```python
from build123d import *
from build123d.topology import SkipClean

# Parameters (mm, degrees)
EXTRUDE_1_DEPTH     = 4
EXTRUDE_START       = -11
SKETCH_3_R          = 9
EXTRUDE_2_DEPTH     = 11
SKETCH_4_R          = 3
CUT_EXTRUDE_1_DEPTH = 50.484262082
HOLE_WIZARD_M4_1_D  = 3.3
SKETCH_10_R         = 6
CUT_EXTRUDE_2_DEPTH = 10
SKETCH_11_R         = 5.5
CUT_EXTRUDE_3_DEPTH = 50.484262082
SCALE1_SCALE        = 2


with BuildPart() as part:
    # 草图1 → 凸台-拉伸1 (new body)
    with BuildSketch(Plane(origin=(0, 0, 0), x_dir=(1, 0, 0), z_dir=(0, 1, 0))):
        with BuildLine():
            Line((-8.109776452, 3.902758754), (-25.406517635, -32.039176982))
            ThreePointArc((-25.406517635, -32.039176982), (-23, -39.837168574), (-15.043482365, -38.022278184))
            Line((-15.043482365, -38.022278184), (0.302963304, -15.526261061))
            Line((0.302963304, -15.526261061), (7.351564548, -25.039059461))
            ThreePointArc((7.351564548, -25.039059461), (12.25592959, -26.282925824), (14.455537758, -21.72642235))
            Line((14.455537758, -21.72642235), (8.752682732, 2.095362733))
            ThreePointArc((8.752682732, 2.095362733), (0.95916746, 8.948742805), (-8.109776452, 3.902758754))
        make_face()
    extrude(amount=EXTRUDE_1_DEPTH)

    # 草图3 → 凸台-拉伸2 (add)
    with SkipClean():  # the faces are left unmerged after this step: merging them gives an invalid solid
        with BuildSketch(Plane(origin=(0, 4, 0), x_dir=(1, 0, 0), z_dir=(0, 1, 0)).offset(EXTRUDE_START)):
            with Locations(Location((0, 0, 0), (0, 0, 154.301222305))):
                Circle(SKETCH_3_R)
        extrude(amount=EXTRUDE_2_DEPTH)

    # 草图4 → 切除-拉伸1 (cut, through all)
    with SkipClean():  # the faces are left unmerged after this step: merging them gives an invalid solid
        with BuildSketch(Plane(origin=(0, 4, 0), x_dir=(1, 0, 0), z_dir=(0, 1, 0))):
            with Locations(Location((-20, -34.641016151, 0), (0, 0, 270))):
                Circle(SKETCH_4_R)
        extrude(amount=-CUT_EXTRUDE_1_DEPTH, mode=Mode.SUBTRACT)

    # M4 螺纹孔1 (through all)
    with Locations(Plane(origin=(0, 4, 0), x_dir=(1, 0, 0), z_dir=(0, 1, 0))):
        with Locations((10.565456544, -22.657694676)):
            Hole(HOLE_WIZARD_M4_1_D / 2)

    # 草图10 → 切除-拉伸2 (cut)
    with SkipClean():  # the faces are left unmerged after this step: merging them gives an invalid solid
        with BuildSketch(Plane(origin=(0, 4, 0), x_dir=(1, 0, 0), z_dir=(0, 1, 0))):
            with Locations(Location((0, 0, 0), (0, 0, 270))):
                Circle(SKETCH_10_R)
        extrude(amount=-CUT_EXTRUDE_2_DEPTH, mode=Mode.SUBTRACT)

    # 草图11 → 切除-拉伸3 (cut, through all)
    with SkipClean():  # the faces are left unmerged after this step: merging them gives an invalid solid
        with BuildSketch(Plane.XZ.offset(7)):
            with Locations(Location((0, 0, 0), (0, 0, 270))):
                Circle(SKETCH_11_R)
        extrude(amount=-CUT_EXTRUDE_3_DEPTH, mode=Mode.SUBTRACT)


with BuildPart() as part_1:
    # Scale1: scaled about (-4.168101576, 0.704724682, 12.285042226)
    add(part.part.scale(SCALE1_SCALE).moved(Location((4.168101576, -0.704724682, -12.285042226))))


solid = part_1.part
```
CAD build for the part. Positions are in the model's coordinates, mm. A direction names the side the tool comes from. Round coordinates to 2 decimals unless told otherwise and drop trailing zeros. Order: outer loops, then holes, each group sorted by start corner. A loop starts at its lowest first (then second) coordinate and runs counter-clockwise, first axis right, second up.
Q1. Slice it at B-B (x = -2). Write the cut outline in (y, z), and give its area (3 significant figures).
Q2. Which spindle directions (+Z, -Z, +X, -X, +Y, -Y) get a long thin tool onto all of the face, cutting with end or side? Do faces 1 (the flat face through (11.724, 3.239, 28.147)), 2 (the flat face through (15, -14.705, -16)), 3 (the flat face through (-6, -12.705, -7)). Say none if no direction does.
Q3. Slice it at D-D (z = 2). Write the cut outline in (x, y).
Q4. Two-plate mould, pull along Z, no slides. Class faces 4 (the flat face through (-8, -0.705, 24)), 5 (the cylindrical face through (-34.03, 3.35, 62.72)), 6 (the flat face through (27.456, 3.239, 7.68)): pulls with the +Z half, pulls with the -Z half, needs draft (parallel to the pull), parting line crosses it, or undercut.
Q5. Wall check: L1, parallel to Y at x = -6, z = 27; L2, parallel to X at y = -3.5, z = -12.5; L3, parallel to X at y = -13, z = -2.5. Give the ranges that are in metal, low to high.
Q6. Slice it at C-C (y = 5.5). Write the cut outline in (x, z), and give its area (3 significant figures).
Q7. Slice it at A-A (z = -11.5). Write the cut outline in (x, y).
Q8. Drop flat-ended pins along their axis: pin 1 (1.5 mm diameter, centred on x = 4, y = 2.5, fed in from +Z); pin 2 (11 mm diameter, centred on x = -35.83, z = 57, fed in from -Y); pin 3 (2 mm diameter, centred on x = 22, z = 20, fed in from -Y). Give the stop position or say it passes through.
Results below:
1. outline: (-14.7, -29.2) - (7.3, -29.2) - (7.3, -22.58) - (-12.7, -22.58) - (-12.7, -21.39) - (-14.7, -21.39) - close; (-14.7, -3.18) - (-12.7, -3.18) - (-12.7, -1.99) - (7.3, -1.99) - (7.3, 28.7) - (-0.7, 28.7) - (-0.7, 4.63) - (-14.7, 4.63) - close
1. area: 488 mm2
2. face 1: +Z, +Y, -Y
2. face 2: +Z, -Z, +X, -X, -Y
2. face 3: +Y
3. outline: (-22.68, -0.7) - (-6.78, -0.7) - (-6.78, -14.7) - (15.12, -14.7) - (15.12, -0.7) - (26.1, -0.7) - (26.1, 7.3) - (-22.68, 7.3) - close
4. face 4: needs draft
4. face 5: undercut
4. face 6: pulls with the -Z half
5. L1: y = -0.7 to 7.3
5. L2: x = -13.83 to -7.83, 16.17 to 22.17
5. L3: x = -10.94 to -0.86, 9.19 to 19.28
6. outline: (-46.64, 51.79) - (-12.05, -20.09) arc R18 ccw to (21.67, -16.48) - (33.08, 31.17) arc R8 ccw to (18.87, 37.79) - (4.77, 18.77) - (-25.92, 63.76) arc R12 ccw to start; hole circle Ø12 at (-35.83, 57); hole circle Ø24 at (4.17, -12.29); hole circle Ø6.6 at (25.3, 33.03)
6. area: 3,310 mm2
7. outline: (-16.19, -0.7) - (-13.81, -0.7) - (-13.81, -14.7) - (-6.8, -14.7) - (-6.8, -12.7) - (-7.81, -12.7) - (-7.81, 7.3) - (-16.19, 7.3) - close; (15.14, -14.7) - (22.15, -14.7) - (22.15, -0.7) - (22.86, -0.7) - (22.86, 7.3) - (16.14, 7.3) - (16.14, -12.7) - (15.14, -12.7) - close
8. pin 1: stops at z = 21
8. pin 2: passes through
8. pin 3: stops at y = -0.7
